Autodesk Inventor part; units mm, degrees
ref_plane "YZ Plane" through (0, 0, 0) normal (1, 0, 0) x (0, 1, 0)
ref_plane "XZ Plane" through (0, 0, 0) normal (0, 1, 0) x (-1, 0, 0)
ref_plane "XY Plane" through (0, 0, 0) normal (0, 0, 1) x (1, 0, 0)
sketch "Sketch1" plane through (0, 0, 0) normal (0, 0, 1) x (1, 0, 0)
  line L0 (-90.5, -90.5) -> (90.5, -90.5)
  line L1 (90.5, -90.5) -> (90.5, 90.5)
  line L2 (90.5, 90.5) -> (-90.5, 90.5)
  line L3 (-90.5, 90.5) -> (-90.5, -90.5)
  line L4 (-90.5, -90.5) -> (90.5, 90.5) construction
  line L5 (90.5, -90.5) -> (-90.5, 90.5) construction
  point P0 (0, 0)
  dimension "d0" = 181
  dimension "d1" = 181
extrude "Extrusion1" add sketch "Sketch1" along normal blind 3
sketch "Sketch3" plane through (0, 0, 3) normal (0, 0, 1) x (1, 0, 0)
  line L0 (-90.5, 90.5) -> (-90.5, -90.5)
  line L1 (-90.5, 82.5) -> (-87.5, 82.5)
  line L2 (-87.5, 82.5) -> (-87.5, 67.5)
  line L3 (-87.5, 67.5) -> (-90.5, 67.5)
  line L4 (-90.5, 67.5) -> (-90.5, 82.5)
  line L5 (-85, 93.5) -> (-90.5, 93.5)
  line L6 (-90.5, 52.5) -> (-87.5, 52.5)
  line L7 (-87.5, 52.5) -> (-87.5, 37.5)
  line L8 (-87.5, 37.5) -> (-90.5, 37.5)
  line L9 (-90.5, 37.5) -> (-90.5, 52.5)
  line L10 (-90.5, 22.5) -> (-87.5, 22.5)
  line L11 (-87.5, 22.5) -> (-87.5, 7.5)
  line L12 (-87.5, 7.5) -> (-90.5, 7.5)
  line L13 (-90.5, 7.5) -> (-90.5, 22.5)
  line L14 (-90.5, -7.5) -> (-87.5, -7.5)
  line L15 (-87.5, -7.5) -> (-87.5, -22.5)
  line L16 (-87.5, -22.5) -> (-90.5, -22.5)
  line L17 (-90.5, -22.5) -> (-90.5, -7.5)
  line L18 (-90.5, -37.5) -> (-87.5, -37.5)
  line L19 (-87.5, -37.5) -> (-87.5, -52.5)
  line L20 (-87.5, -52.5) -> (-90.5, -52.5)
  line L21 (-90.5, -52.5) -> (-90.5, -37.5)
  line L22 (-90.5, -67.5) -> (-87.5, -67.5)
  line L23 (-87.5, -67.5) -> (-87.5, -82.5)
  line L24 (-87.5, -82.5) -> (-90.5, -82.5)
  line L25 (-90.5, -82.5) -> (-90.5, -67.5)
  line L26 (87.5, 82.5) -> (90.5, 82.5)
  line L27 (90.5, 82.5) -> (90.5, 67.5)
  line L28 (90.5, 67.5) -> (87.5, 67.5)
  line L29 (87.5, 67.5) -> (87.5, 82.5)
  line L30 (87.5, 52.5) -> (90.5, 52.5)
  line L31 (90.5, 52.5) -> (90.5, 37.5)
  line L32 (90.5, 37.5) -> (87.5, 37.5)
  line L33 (87.5, 37.5) -> (87.5, 52.5)
  line L34 (87.5, 22.5) -> (90.5, 22.5)
  line L35 (90.5, 22.5) -> (90.5, 7.5)
  line L36 (90.5, 7.5) -> (87.5, 7.5)
  line L37 (87.5, 7.5) -> (87.5, 22.5)
  line L38 (87.5, -7.5) -> (90.5, -7.5)
  line L39 (90.5, -7.5) -> (90.5, -22.5)
  line L40 (90.5, -22.5) -> (87.5, -22.5)
  line L41 (87.5, -22.5) -> (87.5, -7.5)
  line L42 (87.5, -37.5) -> (90.5, -37.5)
  line L43 (90.5, -37.5) -> (90.5, -52.5)
  line L44 (90.5, -52.5) -> (87.5, -52.5)
  line L45 (87.5, -52.5) -> (87.5, -37.5)
  line L46 (87.5, -67.5) -> (90.5, -67.5)
  line L47 (90.5, -67.5) -> (90.5, -82.5)
  line L48 (90.5, -82.5) -> (87.5, -82.5)
  line L49 (87.5, -82.5) -> (87.5, -67.5)
  point P0 (0, 0)
  point P1 (-90.5, -93.5)
  dimension "d27" = 3
  dimension "d28" = 15
  dimension "d29" = 11
  dimension "d32" = 30
  dimension "d35" = 178
extrude "Extrusion3" cut sketch "Sketch3" against normal blind 3
sketch "Sketch4" plane through (0, 0, 3) normal (0, 0, 1) x (1, 0, 0)
  line L0 (80, 93.5) -> (85.5, 93.5)
  line L1 (90.5, 90.5) -> (-90.5, 90.5)
  line L2 (85.5, 93.5) -> (90.5, 93.5)
  line L3 (90.5, 93.5) -> (90.5, 90.5)
  line L4 (90.5, 90.5) -> (85.5, 90.5)
  line L5 (85.5, 90.5) -> (85.5, 93.5)
  line L6 (-90.5, -90.5) -> (90.5, -90.5)
  line L7 (85.5, -90.5) -> (90.5, -90.5)
  line L8 (90.5, -90.5) -> (90.5, -93.5)
  line L9 (90.5, -93.5) -> (85.5, -93.5)
  line L10 (85.5, -93.5) -> (85.5, -90.5)
  point P0 (0, 0)
  point P1 (85.5, 90.5)
  dimension "d40" = 184
extrude "Extrusion4" add sketch "Sketch4" against normal blind 3
sketch "Sketch6" plane through (0, 0, 0) normal (0, 0, -1) x (-1, 0, 0)
  line L0 (-90.5, 82.5) -> (-90.5, 93.5)
  line L1 (-90.5, 93.5) -> (-75, 93.5)
  line L2 (-75, 93.5) -> (-75, -93.5)
  line L3 (-75, -93.5) -> (-90.5, -93.5)
  line L4 (-90.5, -93.5) -> (-90.5, 93.5)
  line L5 (85, 93.5) -> (90.5, 93.5)
  line L6 (90.5, 93.5) -> (46.5, 93.5)
  line L7 (46.5, 93.5) -> (46.5, -93.5)
  line L8 (46.5, -93.5) -> (90.5, -93.5)
  line L9 (90.5, -93.5) -> (90.5, 93.5)
  point P0 (0, 0)
  dimension "d47" = 15.5
  dimension "d48" = 44
  dimension "d49" = 187
  dimension "d50" = 187
extrude "Extrusion6" cut sketch "Sketch6" against normal blind 10
sketch "Sketch7" plane through (0, 0, 3) normal (0, 0, 1) x (1, 0, 0)
  circle A0 centre (-38.5, 73.5) radius 2
  circle A1 centre (-38.5, 63.5) radius 2
  circle A2 centre (-38.5, 5) radius 2
  circle A3 centre (-38.5, -5) radius 2
  circle A4 centre (-38.5, -63.5) radius 2
  circle A5 centre (-38.5, -73.5) radius 2
  line L0 (-40, 93.5) -> (-25, 93.5)
  line L1 (-25, -93.5) -> (-40, -93.5)
  line L2 (-46.5, 90.5) -> (-46.5, -90.5)
  point P0 (0, 0)
  dimension "d53" = 4
  dimension "d54" = 4
  dimension "d55" = 4
  dimension "d56" = 4
  dimension "d57" = 4
  dimension "d58" = 4
  dimension "d59" = 0
  dimension "d60" = 0
  dimension "d61" = 0
  dimension "d62" = 10
  dimension "d63" = 10
  dimension "d64" = 10
  dimension "d65" = 20
  dimension "d66" = 20
  dimension "d67" = 8
  dimension "d68" = 8
  dimension "d69" = 8
  dimension "d70" = 5
extrude "Extrusion7" cut sketch "Sketch7" against normal blind 10
sketch "Sketch8" plane through (0, 0, 3) normal (0, 0, 1) x (1, 0, 0)
  line L0 (-46.5, 90.5) -> (75, 90.5)
  line L1 (75, 90.5) -> (75, 93.5)
  line L2 (75, 93.5) -> (-46.5, 93.5)
  line L3 (-46.5, 93.5) -> (-46.5, 90.5)
  line L4 (-46.5, -93.5) -> (75, -93.5)
  line L5 (75, -93.5) -> (75, -90.5)
  line L6 (75, -90.5) -> (-46.5, -90.5)
  line L7 (-46.5, -90.5) -> (-46.5, -93.5)
  point P0 (0, 0)
  dimension "d81" = 121.5
  dimension "d82" = 3
  dimension "d85" = 184
extrude "Extrusion8" add sketch "Sketch8" against normal blind 3
sketch "Sketch9" plane through (0, 0, 3) normal (0, 0, 1) x (1, 0, 0)
  line L0 (21.75, 15) -> (69.75, 15) construction
  line L1 (69.75, 15) -> (69.75, -15) construction
  line L2 (69.75, -15) -> (21.75, -15) construction
  line L3 (21.75, -15) -> (21.75, 15) construction
  line L4 (21.75, 15) -> (69.75, -15) construction
  line L5 (69.75, 15) -> (21.75, -15) construction
  line L6 (75, -93.5) -> (75, 93.5)
  circle A0 centre (21.75, 15) radius 2
  circle A1 centre (69.75, 15) radius 2
  circle A2 centre (69.75, -15) radius 2
  circle A3 centre (21.75, -15) radius 2
  point P0 (0, 0)
  point P1 (45.75, 0)
  dimension "d92" = 48
  dimension "d93" = 30
  dimension "d94" = 0
  dimension "d95" = 5.25
  dimension "d96" = 4
  dimension "d97" = 4
  dimension "d98" = 4
  dimension "d99" = 4
extrude "Extrusion9" cut sketch "Sketch9" against normal blind 3
equation "\"d54\" = d53"
equation "\"d55\" = d53"
equation "\"d56\" = d55"
equation "\"d57\" = d56"
equation "\"d58\" = d57"
equation "\"d63\" = d62"
equation "\"d64\" = d62"
equation "\"d68\" = d67"
equation "\"d69\" = d67"
equation "\"BendRadius\" = Thickness"
equation "\"BendReliefWidth\" = Thickness"
equation "\"BendReliefDepth\" = 0.5 * Thickness"
equation "\"CornerReliefSize\" = 4 * Thickness"
equation "\"MinimumRemnant\" = 2 * Thickness"
equation "\"TransitionRadius\" = BendRadius"
equation "\"JacobiRadiusSize\" = BendRadius"
equation "\"GapSize\" = Thickness"
properties part number "11 deur plaat"
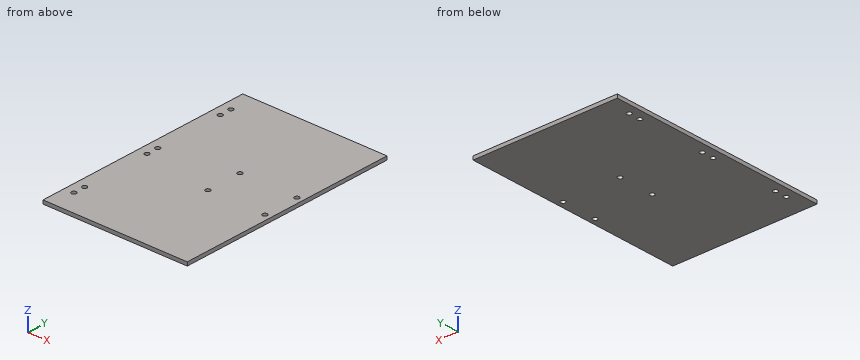
For this review, take the finished solid that the model builds, in its own axes (mm). Round coordinates to 2 decimals unless told otherwise and drop trailing zeros. Loops run counter-clockwise (first coordinate to the right, second up) from the corner with the lowest first, then second, coordinate; pieces in that order, holes last.
Q1. Insertion check: pin 1 Ø3.5 at (x, y) = (-38.5, 63.5) entering from -Z; pin 2 Ø5 at (x, y) = (34.5, 12.5) entering from -Z. Each pin has a flat end and moves straight along its axis. Give the tip position at first contact, or say it passes through.
Result sheet:
pin 1: passes through
pin 2: stops at z = 0
Q2. To check wall thickness, follow line 1 along Y through (x, z) = (21.5, 1.3); line 2 along X through (y, z) = (-6, 1.7). State the ranges of each line that lie inside material, in increasing order.
Result sheet:
line 1: y = -93.5 to -16.98, -13.02 to 13.02, 16.98 to 93.5
line 2: x = -46.5 to -40.23, -36.77 to 75
Q3. Add section B-B on x = 69.75. Write out the cut boundary in (y, z), plus the area to 3 significant figures.
Result sheet:
outline: (-93.5, 0) - (-17, 0) - (-17, 3) - (-93.5, 3) - close; (-13, 0) - (13, 0) - (13, 3) - (-13, 3) - close; (17, 0) - (93.5, 0) - (93.5, 3) - (17, 3) - close
area: 537 mm2
Q4. Add section C-C on x = -38.5. Write out the cut boundary in (y, z).
Result sheet:
outline: (-93.5, 0) - (-75.5, 0) - (-75.5, 3) - (-93.5, 3) - close; (-71.5, 0) - (-65.5, 0) - (-65.5, 3) - (-71.5, 3) - close; (-61.5, 0) - (-7, 0) - (-7, 3) - (-61.5, 3) - close; (-3, 0) - (3, 0) - (3, 3) - (-3, 3) - close; (7, 0) - (61.5, 0) - (61.5, 3) - (7, 3) - close; (65.5, 0) - (71.5, 0) - (71.5, 3) - (65.5, 3) - close; (75.5, 0) - (93.5, 0) - (93.5, 3) - (75.5, 3) - close
Q5. Add section A-A on y = 15. Write out the cut boundary in (x, z), plus the area to 4 significant figures.
Result sheet:
outline: (-46.5, 0) - (19.75, 0) - (19.75, 3) - (-46.5, 3) - close; (23.75, 0) - (67.75, 0) - (67.75, 3) - (23.75, 3) - close; (71.75, 0) - (75, 0) - (75, 3) - (71.75, 3) - close
area: 340.5 mm2
Q6. Add section D-D on y = -73.5. Write out the cut boundary in (x, z).
Result sheet:
outline: (-46.5, 0) - (-40.5, 0) - (-40.5, 3) - (-46.5, 3) - close; (-36.5, 0) - (75, 0) - (75, 3) - (-36.5, 3) - close
